```python
from build123d import *

# Parameters (mm, degrees)
SKETCH2_R               = 3.3655
CUT_EXTRUDE1_DEPTH      = 26.4
CUT_EXTRUDE1_DEPTH_BACK = 26.4
FILLET1_R               = 1.6002
CHAMFER1_SIZE           = 0.4699
CHAMFER2_SIZE           = 0.635


with BuildPart() as part:
    # Sketch1 → Revolve1 (revolve)
    with BuildSketch(Plane.XY, mode=Mode.PRIVATE) as revolve1_sk:
        with BuildLine():
            Line((25.4, 0), (25.4, 24.13))
            Line((25.4, 24.13), (12.7, 63.600954744))
            ThreePointArc((12.7, 63.600954744), (24.534515988, 92.172003746), (0, 110.998))
            Line((0, 110.998), (0, 28.575))
            Line((0, 28.575), (4.1656, 26.072055005))
            Line((4.1656, 26.072055005), (4.1656, 0.508))
            Line((4.1656, 0.508), (17.145, 0.508))
            Line((17.145, 0.508), (17.145, 0))
            Line((17.145, 0), (25.4, 0))
        make_face()
    revolve(revolve1_sk.sketch.rotate(Axis((0, 0, 0), (0, 1, 0)), 90), axis=Axis((0, 0, 0), (0, 1, 0)))  # turned: the seam where the file's is

    # Sketch2 → Cut-Extrude1 (cut, two sides)
    with BuildSketch(Plane.XY) as cut_extrude1_sk:
        with Locations(Location((0, 35.8775, 0), (0, 0, 90.000000009))):  # turned: the seam where the file's is
            Circle(SKETCH2_R)
    extrude(amount=CUT_EXTRUDE1_DEPTH, mode=Mode.SUBTRACT)
    extrude(cut_extrude1_sk.sketch, amount=-CUT_EXTRUDE1_DEPTH_BACK, mode=Mode.SUBTRACT)

    # Fillet1
    fillet1_edges = [part.edges().sort_by_distance(p)[0] for p in [
        (0, 24.13, 25.4),
    ]]
    fillet(fillet1_edges, radius=FILLET1_R)

    # Chamfer1
    chamfer1_edges = [part.edges().sort_by_distance(p)[0] for p in [
        (0, 0, 17.145),
    ]]
    chamfer(chamfer1_edges, length=CHAMFER1_SIZE)

    # Chamfer2
    chamfer2_edges = [part.edges().sort_by_distance(p)[0] for p in [
        (0, 0.508, 4.1656),
    ]]
    chamfer(chamfer2_edges, length=CHAMFER2_SIZE)


solid = part.part
```
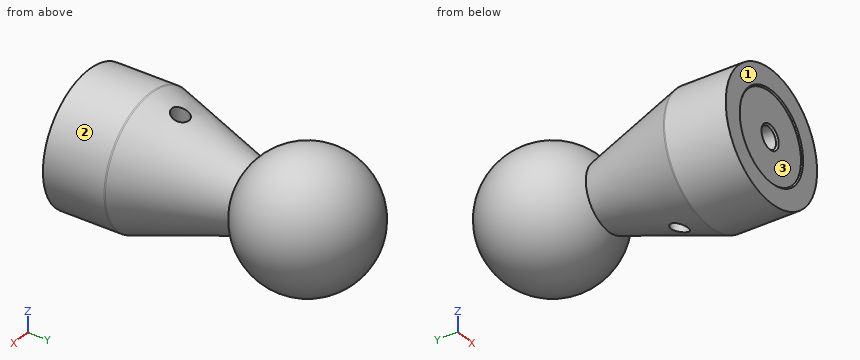
For this review, take the finished solid that the model builds, in its own axes (mm). Face numbers are marked on the shaded views. Round coordinates to 2 decimals unless told otherwise and drop trailing zeros. Write each loop counter-clockwise with the first axis right and the second up, starting at its lowest first coordinate (ties: lowest second). Pieces come first, ordered by that corner, then holes. Notation, with made-up numbers: M -0.75,-34.75 L 38.25,-34.75 A20 ccw 38.25,1.25 Z; hole C -19.5,60 d8. An arc over 180 degrees is marked long. One line per item, written item: value. Start each with the question number.
(1) We need section A-A (y = 7). Give the boundary of the cut face in (x, z).
(2) We need section C-C (y = 96). Give the boundary of the cut face in (x, z), and give its area (3 significant figures).
(3) Insertion check: pin 1 (10.5 mm diameter, centred on x = -6.5, z = 3, fed in from -Y); pin 2 (4 mm diameter, centred on x = 9.5, y = 93, fed in from -Z); pin 3 (6 mm diameter, centred on x = 1, y = 64, fed in from +Z). Each pin has a flat end and moves straight along its axis. Give the tip position at first contact, or say it passes through.
(4) We need section B-B (y = 57). Give the boundary of the cut face in (x, z), and give its area (3 significant figures).
(5) The part is to be moulded in two halves that separate along X. For the marked faces 1, 2 and 3, say which applies: released by +X, released by -X, zero draft, split by the parting line, or undercut.
(6) Wall thickness on line 1 (Y direction, x = 0, z = 12); line 2 (X direction, y = 0.55, z = 0); line 3 (X direction, y = 37, z = 8.5): over which ranges is each line inside the solid? List them lowest first.
Result:
1. outline: C 0,0 d50.8; hole C 0,0 d8.33
2. outline: C 0,0 d46.34
2. area: 1,690 mm²
3. pin 1: y = 0.51
3. pin 2: z = -23.33
3. pin 3: z = 17.27
4. outline: C 0,0 d29.65
4. area: 690 mm²
5. face 1: zero draft
5. face 2: split by the parting line
5. face 3: undercut
6. line 1: 0.51 to 32.51, 39.24 to 107.98
6. line 2: -25.4 to -4.76, 4.76 to 25.4
6. line 3: -19.49 to -3.17, 3.17 to 19.49
